Work out the finished part from the listing and answer in its coordinate system (mm). Face numbers are marked on the shaded views. A direction names the side the tool comes from. Round coordinates to 2 decimals unless told otherwise and drop trailing zeros. Order: outer loops, then holes, each group sorted by start corner. A loop starts at its lowest first (then second) coordinate and runs counter-clockwise, first axis right, second up. Notation, with made-up numbers: (21.25, 48.5) -> (54.25, 48.5) arc R17 cw to (54.25, 56.5) -> close; hole circle Ø2 at (3.25, -14.5). An arc over 180 degrees is marked (long way). Use a Markdown table: item, result. Add a question column.
Item 1: For a pull along X with two mould halves and no side action, classify the marked faces 3, 4 and 5 as +X half, -X half, draft (parallel to the pull), parting line (faces both ways), or undercut.
Item 2: A cutting plane is placed at D-D, the plane x = 5. Determine the outline of the cut face in (y, z) (3 decimals).
Item 3: A tool of negligible diameter and unlimited length cuts with its end or side. For the marked faces 1 and 2, from which of +Z, -Z, +X, -X, +Y, -Y can it reach the whole face along a straight path? Write none if from no direction.
Item 4: Find the intervals of material crossed by L1, parallel to Z at x = 17, y = 0 (3 decimals); L2, parallel to Z at x = -17, y = 0 (3 decimals); L3, parallel to Y at x = -12.5, z = -19.5 (3 decimals), in increasing order. Write a range as [from, to].
Item 5: A flat-ended cylindrical pin translates along its axis: P1, Ø10, axis at x = -3.5, y = 14.5, coming from the +Z side (3 decimals). Find the tip coordinate at first contact, or state that the pin passes through.
Item 6: A cutting plane is placed at B-B, the plane z = 105. Determine the outline of the cut face in (x, y) (3 decimals).
Item 7: A cutting plane is placed at C-C, the plane y = -10. Determine the outline of the cut face in (x, z) (3 decimals).
Item 8: A cutting plane is placed at A-A, the plane y = 0. Give the number of separate pieces and of enclosed holes in the cut face, plus the area to 3 significant figures.
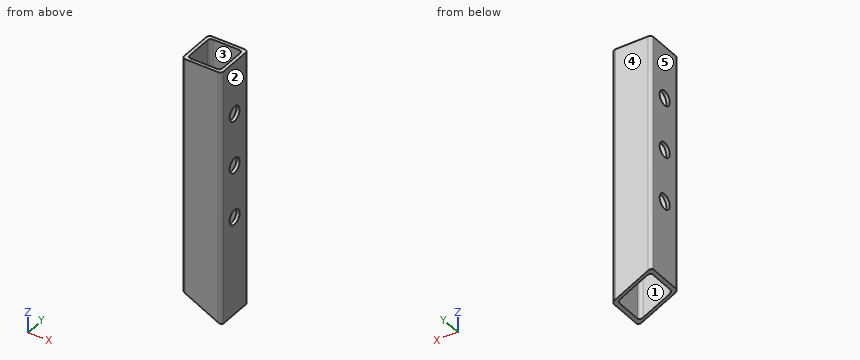
from build123d import *

# Parameters (mm, degrees)
F0_W     = 38.1
F0_H     = 38.1
F1_DEPTH = 123.825
F2_T     = -3.175
F3_R     = 7.14375
F4_DEPTH = 38.101
F6_DEPTH = 38.101
F7_R     = 3.175


with BuildPart() as f1:
    # F0 (on Top) → F1 (new body, symmetric)
    with BuildSketch(Plane.XY):
        Rectangle(F0_W, F0_H)
    extrude(amount=F1_DEPTH, both=True)

    # F2
    f2_openings = [f1.faces().sort_by_distance(p)[0] for p in [
        (0, 0, 123.825),
        (0, 0, -123.825),
    ]]
    offset(amount=F2_T, openings=f2_openings)

    # F3 (on face) → F4 (cut, through all)
    with BuildSketch(Plane.YZ.offset(19.05)):
        with Locations((0, 73.025)):
            Circle(F3_R)
        with Locations((0, 22.225)):
            Circle(F3_R)
        with Locations((0, -28.575)):
            Circle(F3_R)
    extrude(amount=-F4_DEPTH, mode=Mode.SUBTRACT)

    # F5 (on face) → F6 (cut, through all)
    with BuildSketch(Plane.XZ.offset(19.05)):
        Polygon((-19.05, -123.825), (19.05, -123.825), (-19.05, -104.7708862961), align=None)
    extrude(amount=-F6_DEPTH, mode=Mode.SUBTRACT)

    # F7
    f7_edges = [f1.edges().sort_by_distance(p)[0] for p in [
        (-19.05, -19.05, 9.527057),
        (19.05, 19.05, 0),
        (19.05, -19.05, 0),
        (-19.05, 19.05, 9.527057),
        (-15.875, -15.875, 8.733135),
        (-15.875, 15.875, 8.733135),
        (15.875, 15.875, 0.793921),
        (15.875, -15.875, 0.793921),
    ]]
    fillet(f7_edges, radius=F7_R)


solid = f1.part
Reported:
| question | item | result |
|---|---|---|
| 1 | face 3 | undercut |
| 1 | face 4 | draft |
| 1 | face 5 | -X half |
| 2 | outline | (-19.05, -116.798) -> (-15.875, -116.798) -> (-15.875, 123.825) -> (-19.05, 123.825) -> close; (15.875, -116.798) -> (19.05, -116.798) -> (19.05, 123.825) -> (15.875, 123.825) -> close |
| 3 | face 1 | +Z, -Z |
| 3 | face 2 | +Z, -Z, +X, +Y, -Y |
| 4 | L1 | [-122.8, -35.719], [-21.431, 15.081], [29.369, 65.881], [80.169, 123.825] |
| 4 | L2 | [-105.796, -35.719], [-21.431, 15.081], [29.369, 65.881], [80.169, 123.825] |
| 4 | L3 | [-19.05, -15.875], [15.875, 19.05] |
| 5 | P1 | z = 123.825 |
| 6 | outline | (-19.05, -15.875) arc R3.175 ccw to (-15.875, -19.05) -> (15.875, -19.05) arc R3.175 ccw to (19.05, -15.875) -> (19.05, 15.875) arc R3.175 ccw to (15.875, 19.05) -> (-15.875, 19.05) arc R3.175 ccw to (-19.05, 15.875) -> close; hole (-15.875, -12.7) arc R3.175 ccw to (-12.7, -15.875) -> (12.7, -15.875) arc R3.175 ccw to (15.875, -12.7) -> (15.875, 12.7) arc R3.175 ccw to (12.7, 15.875) -> (-12.7, 15.875) arc R3.175 ccw to (-15.875, 12.7) -> close |
| 7 | outline | (-19.05, -104.771) -> (-15.875, -106.359) -> (-15.875, 123.825) -> (-19.05, 123.825) -> close; (15.875, -122.237) -> (19.05, -123.825) -> (19.05, 123.825) -> (15.875, 123.825) -> close |
| 8 | separate pieces | 8 |
| 8 | enclosed holes | 0 |
| 8 | area | 1,240 mm² |
